```python
from build123d import *

# Parameters (mm, degrees)
F0_W           = 280
F0_H           = 88
F1_DEPTH       = 5
F6_D           = 3.2
F6_DEPTH       = 17.25
F6_TIP         = 0.9613769904
F6_ON_F5_D     = 3.2
F6_ON_F5_DEPTH = 17.25
F6_ON_F5_TIP   = 0.9613769904
F6_ON_F3_D     = 3.2
F6_ON_F3_DEPTH = 17.25
F6_ON_F3_TIP   = 0.9613769904
F6_ON_F2_D     = 3.2
F6_ON_F2_DEPTH = 17.25
F6_ON_F2_TIP   = 0.9613769904
F8_D           = 4.4
F8_CBORE_D     = 8
F8_CBORE_DEPTH = 4
F10_D          = 2.4


with BuildPart() as f1:
    # F0 (on Front) → F1 (new body, symmetric)
    with BuildSketch(Plane.XZ):
        Rectangle(F0_W, F0_H)
    extrude(amount=F1_DEPTH, both=True)

    # F6
    with Locations(Plane.XY.offset(44)):
        with Locations((110, 0), (-110, 0)):
            Hole(F6_D / 2, depth=F6_DEPTH)
            with Locations((0, 0, -(F6_DEPTH + F6_TIP / 2))):  # 118° drill point
                Cone(0, F6_D / 2, F6_TIP, mode=Mode.SUBTRACT)

    # F6 on F5
    with Locations(Plane(origin=(0, 0, -44), x_dir=(1, 0, 0), z_dir=(0, 0, -1))):
        with Locations((-110, 0), (110, 0)):
            Hole(F6_ON_F5_D / 2, depth=F6_ON_F5_DEPTH)
            with Locations((0, 0, -(F6_ON_F5_DEPTH + F6_ON_F5_TIP / 2))):  # 118° drill point
                Cone(0, F6_ON_F5_D / 2, F6_ON_F5_TIP, mode=Mode.SUBTRACT)

    # F6 on F3
    with Locations(Plane.YZ.offset(140)):
        with Locations((0, -24), (0, 24)):
            Hole(F6_ON_F3_D / 2, depth=F6_ON_F3_DEPTH)
            with Locations((0, 0, -(F6_ON_F3_DEPTH + F6_ON_F3_TIP / 2))):  # 118° drill point
                Cone(0, F6_ON_F3_D / 2, F6_ON_F3_TIP, mode=Mode.SUBTRACT)

    # F6 on F2
    with Locations(Plane(origin=(-140, 0, 0), x_dir=(0, -1, 0), z_dir=(-1, 0, 0))):
        with Locations((0, -24), (0, 24)):
            Hole(F6_ON_F2_D / 2, depth=F6_ON_F2_DEPTH)
            with Locations((0, 0, -(F6_ON_F2_DEPTH + F6_ON_F2_TIP / 2))):  # 118° drill point
                Cone(0, F6_ON_F2_D / 2, F6_ON_F2_TIP, mode=Mode.SUBTRACT)

    # F8 (through all)
    with Locations(Plane.XZ.offset(5)):
        with Locations((-39.25, 5), (39.25, 5), (-39.25, -5), (39.25, -5)):
            CounterBoreHole(F8_D / 2, F8_CBORE_D / 2, F8_CBORE_DEPTH)

    # F10 (through all)
    with Locations(Plane.XZ.offset(5)):
        with Locations((85, 38), (55, 38)):
            Hole(F10_D / 2)


solid = f1.part
```
Source: CAD feature listing. Evaluate the final solid. Frame: model axes, mm. A direction names the side the tool comes from. Round coordinates to 2 decimals unless told otherwise and drop trailing zeros.
1. Mould query, pull axis X, two halves, no side actions, for faces 3 (the flat face through (140, 0, -1)), 4 (the flat face through (-38, -1, -7)), 5 (the flat face through (41, -1, -7)), 6 (the flat face through (-2, 0, 44)). Classes: released by +X, released by -X, zero draft, split by the parting line, or undercut.
2. Contact query for flat-ended pins moving along their axis: pin 1 (3.5 mm diameter, centred on x = 39.25, z = 5, fed in from +Y); pin 2 (6.5 mm diameter, centred on x = 39, z = 5.5, fed in from -Y); pin 3 (4 mm diameter, centred on y = 0, z = -24, fed in from +X); pin 4 (2.5 mm diameter, centred on x = -110, y = 0, fed in from +Z). Output: stop coordinate, or through.
3. Access query for faces 1 (the flat face through (41, -1, 3)), 2 (the flat face through (-140, 0, -1)). Directions: +Z, -Z, +X, -X, +Y, -Y. A direction counts if a zero-diameter tool reaches every point of the face in a straight line with its end or side. Return the directions, or none.
4. Ray query, L1, parallel to X at y = -2.75, z = 5.5; L2, parallel to Z at x = -128.25, y = 0; L3, parallel to Y at x = 110, z = 38.5. Return the intervals inside material, ascending.
Answers below:
1. face 3: released by +X
1. face 4: undercut
1. face 5: undercut
1. face 6: zero draft
2. pin 1: passes through
2. pin 2: stops at y = -1
2. pin 3: stops at x = 140
2. pin 4: stops at z = 26.54
3. face 1: -Y
3. face 2: +Z, -Z, -X, +Y, -Y
4. L1: x = -140 to -43.22, -35.28 to 35.28, 43.22 to 140
4. L2: z = -44 to -25.6, -22.4 to 22.4, 25.6 to 44
4. L3: y = -5 to -1.6, 1.6 to 5
